Geometry: see drawing. Coordinates: mm, zero at the bounding-box minimum. A direction names the side the tool comes from. Coordinates: 2 decimals unless noted, no trailing zeros. Loops run counter-clockwise (first coordinate to the right, second up) from the corner with the lowest first, then second, coordinate; pieces in that order, holes last. Notation, with made-up numbers: (-33, -9) - (11, -9) arc R20 cw to (11, 16) - close; hole circle Ø8 at (33.5, 43.5). An arc over 180 degrees is marked (long way). Use a Markdown table: item, result. Add a question column.
1. Section query C-C on z = 8.25. Return the cut outline in (x, y) (3 decimals).
2. Access query for the marked faces 1 and 2. Directions: +Z, -Z, +X, -X, +Y, -Y. A direction counts if a zero-diameter tool reaches every point of the face in a straight line with its end or side. Return the directions, or none.
3. Contact query for flat-ended pins moving along their axis: P1, Ø1, axis at x = 8.5, z = 4.5, coming from the -Y side; P2, Ø3, axis at x = 1.5, z = 7, coming from the +Y side; P3, Ø1, axis at y = 8.5, z = 5.5, coming from the +X side. Output: stop coordinate, or through.
4. Section query A-A on y = 5. Return the cut outline in (x, z) (3 decimals), then the cut area to 3 significant figures.
5. Section query D-D on z = 11.75. Return the cut outline in (x, y).
6. Ray query, L1, parallel to Y at x = 5, z = 6.25 (3 decimals); L2, parallel to Z at x = 6.75, y = 8.25; L3, parallel to Z at x = 7.75, y = 3. Return the intervals inside material, ascending. Write a range as [from, to].
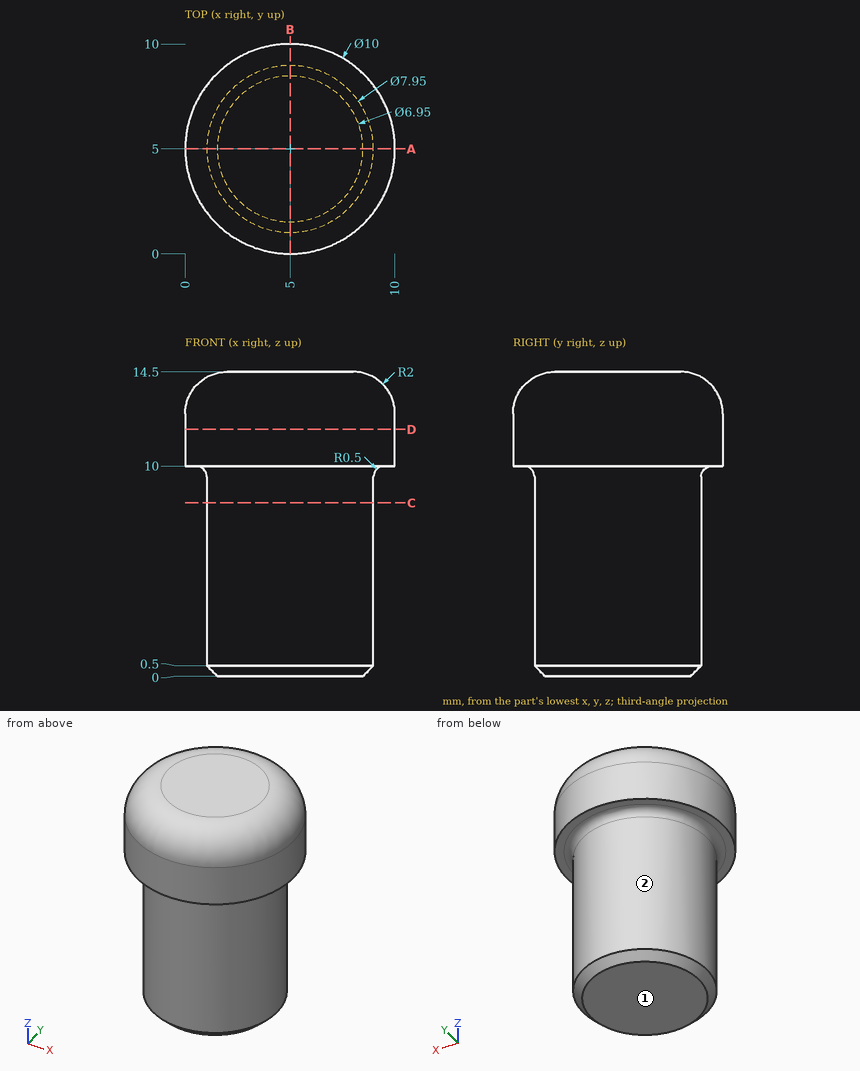
Resolved:
| question | item | result |
|---|---|---|
| 1 | outline | circle Ø7.95 at (5, 5) |
| 2 | face 1 | -Z, +X, -X, +Y, -Y |
| 2 | face 2 | -Z |
| 3 | P1 | y = 2.39 |
| 3 | P2 | y = 8.44 |
| 3 | P3 | x = 7.61 |
| 4 | outline | (0, 10) - (0.525, 10) arc R0.5 cw to (1.025, 9.5) - (1.025, 0.5) - (1.525, 0) - (8.475, 0) - (8.975, 0.5) - (8.975, 9.5) arc R0.5 cw to (9.475, 10) - (10, 10) - (10, 12.5) arc R2 ccw to (8, 14.5) - (2, 14.5) arc R2 ccw to (0, 12.5) - close |
| 4 | area | 123 mm² |
| 5 | outline | circle Ø10 at (5, 5) |
| 6 | L1 | [1.025, 8.975] |
| 6 | L2 | [0.22, 14.38] |
| 6 | L3 | [0, 14.46] |
